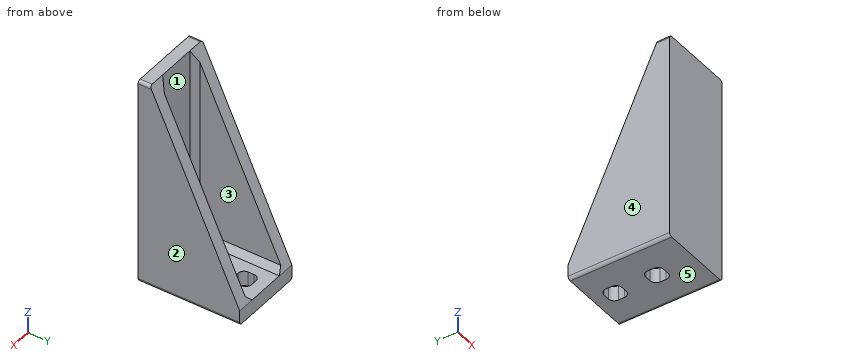
from build123d import *

# Parameters (mm, degrees)
ESBO_O1_W               = 25
ESBO_O1_H               = 70
BASE_DEPTH              = 4
ESBO_O2_W               = 25
ESBO_O2_H               = 5
PAREDE_DO_FUNDO_DEPTH   = 30
PAREDES_START           = -12.5
PAREDES_LATERAIS_DEPTH  = 25
ESBO_O3_W               = 17
ESBO_O3_H               = 30
CORTE_NAS_PAREDES_DEPTH = 65
CHANFRO3_SIZE           = 2
CHANFRO4_SIZE           = 2
CHANFRO5_SIZE           = 2
CHANFRO6_SIZE           = 2
CHANFRO7_SIZE           = 2
PARAFUSO_DEPTH          = 45
FILETE1_R               = 1
FILETE2_R               = 1
FILETE3_R               = 1
FILETE4_R               = 1


with BuildPart() as part:
    # Esboço1 → Base (new body)
    with BuildSketch(Plane(origin=(0, 0, 0), x_dir=(1, 0, 0), z_dir=(0, 1, 0))):
        Rectangle(ESBO_O1_W, ESBO_O1_H)
    extrude(amount=BASE_DEPTH)

    # Esboço2 → Parede do fundo (add)
    with BuildSketch(Plane(origin=(0, 4, 0), x_dir=(1, 0, 0), z_dir=(0, 1, 0))):
        with Locations((0, 32.5)):
            Rectangle(ESBO_O2_W, ESBO_O2_H)
    extrude(amount=PAREDE_DO_FUNDO_DEPTH)

    # Paredes Laterais: read off the stored shape, not the designer's step
    # Paredes Laterais outline → Paredes Laterais (add)
    with BuildSketch(Plane.YZ.offset(PAREDES_START)):
        Polygon((34, -30), (4, 35), (4, -30), align=None)
    extrude(amount=PAREDES_LATERAIS_DEPTH)

    # Esboço3 → Corte nas Paredes (cut)
    with BuildSketch(Plane.XY.offset(35)):
        with Locations((0, 19)):
            Rectangle(ESBO_O3_W, ESBO_O3_H)
    extrude(amount=-CORTE_NAS_PAREDES_DEPTH, mode=Mode.SUBTRACT)

    # Chanfro3
    chanfro3_edges = [part.edges().sort_by_distance(p)[0] for p in [
        (-8.5, 4, 2.5),
    ]]
    chamfer(chanfro3_edges, length=CHANFRO3_SIZE)

    # Chanfro4
    chanfro4_edges = [part.edges().sort_by_distance(p)[0] for p in [
        (8.5, 4, 2.5),
    ]]
    chamfer(chanfro4_edges, length=CHANFRO4_SIZE)

    # Chanfro5
    chanfro5_edges = [part.edges().sort_by_distance(p)[0] for p in [
        (0, 4, -30),
    ]]
    chamfer(chanfro5_edges, length=CHANFRO5_SIZE)

    # Chanfro6
    chanfro6_edges = [part.edges().sort_by_distance(p)[0] for p in [
        (-8.5, 20, -30),
    ]]
    chamfer(chanfro6_edges, length=CHANFRO6_SIZE)

    # Chanfro7
    chanfro7_edges = [part.edges().sort_by_distance(p)[0] for p in [
        (8.5, 20, -30),
    ]]
    chamfer(chanfro7_edges, length=CHANFRO7_SIZE)

    # Esboço4 → Parafuso (cut)
    with BuildSketch(Plane(origin=(0, 0, -35), x_dir=(-1, 0, 0), z_dir=(0, 0, -1))):
        with BuildLine():
            Line((-1, 16), (1, 16))
            ThreePointArc((1, 16), (2.414213562, 15.414213562), (3, 14))
            Line((3, 14), (3, 12))
            ThreePointArc((3, 12), (2.414213562, 10.585786438), (1, 10))
            Line((1, 10), (-1, 10))
            ThreePointArc((-1, 10), (-2.414213562, 10.585786438), (-3, 12))
            Line((-3, 12), (-3, 14))
            ThreePointArc((-3, 14), (-2.414213562, 15.414213562), (-1, 16))
        make_face()
        with BuildLine():
            Line((-3, 26), (-3, 28))
            ThreePointArc((-3, 28), (-2.414213562, 29.414213562), (-1, 30))
            Line((-1, 30), (1, 30))
            ThreePointArc((1, 30), (2.414213562, 29.414213562), (3, 28))
            Line((3, 28), (3, 26))
            ThreePointArc((3, 26), (2.414213562, 24.585786438), (1, 24))
            Line((1, 24), (-1, 24))
            ThreePointArc((-1, 24), (-2.414213562, 24.585786438), (-3, 26))
        make_face()
    extrude(amount=-PARAFUSO_DEPTH, mode=Mode.SUBTRACT)

    # Filete1
    filete1_edges = [part.edges().sort_by_distance(p)[0] for p in [
        (12.5, 17, -35),
    ]]
    fillet(filete1_edges, radius=FILETE1_R)

    # Filete2
    filete2_edges = [part.edges().sort_by_distance(p)[0] for p in [
        (-12.5, 17, -35),
    ]]
    fillet(filete2_edges, radius=FILETE2_R)

    # Filete3
    filete3_edges = [part.edges().sort_by_distance(p)[0] for p in [
        (12.5, 2, 35),
    ]]
    fillet(filete3_edges, radius=FILETE3_R)

    # Filete4
    filete4_edges = [part.edges().sort_by_distance(p)[0] for p in [
        (-12.5, 2, 35),
    ]]
    fillet(filete4_edges, radius=FILETE4_R)


solid = part.part
Geometry: final body of the model. Coordinates: model frame, mm. Face numbers are marked on the shaded views. A direction names the side the tool comes from. Round coordinates to 2 decimals unless told otherwise and drop trailing zeros. Loops run counter-clockwise (first coordinate to the right, second up) from the corner with the lowest first, then second, coordinate; pieces in that order, holes last.
Q1. Section A-A on x = -1.75. Return loops of the section in (y, z), plus the area to 3 significant figures.
Q2. Section D-D on z = -20.5. Return loops of the section in (x, y), plus the area to 3 significant figures.
Q3. Pull-direction query (X, two-part tool) for the marked faces 3, 4 and 5; classes: released by +X, released by -X, zero draft, split by the parting line, or undercut.
Q4. Section C-C on x = 9.75. Return loops of the section in (y, z).
Q5. Section B-B on y = 8.5. Return loops of the section in (x, z).
Q6. Material intervals for L1, parallel to Y at x = 1.25, z = -31; L2, parallel to X at y = 13, z = -1; L3, parallel to Y at x = 5.25, z = -24, sorted ascending.
Q7. Access query for the marked faces 1 and 2. Directions: +Z, -Z, +X, -X, +Y, -Y. A direction counts if a zero-diameter tool reaches every point of the face in a straight line with its end or side. Return the directions, or none.
Q8. Pin query (flat end, axial travel): P1, Ø12, axis at x = 7.5, y = 26, coming from the +Z side; P2, Ø1.6, axis at x = 0.5, z = -31.5, coming from the -Y side; P3, Ø2, axis at x = -7, y = 7, coming from the +Z side; P4, Ø3, axis at x = 3.5, z = -4.5, coming from the +Y side. Return the tip coordinate at first contact, or that it passes through.
Evaluation:
1. outline: (0, -35) - (10.15, -35) - (10.15, -30) - (6, -30) - (4, -28) - (4, 35) - (0, 35) - close; (15.85, -35) - (24.15, -35) - (24.15, -30) - (15.85, -30) - close; (29.85, -35) - (34, -35) - (34, -30) - (29.85, -30) - close
1. area: 375 mm2
2. outline: (-12.5, 0) - (12.5, 0) - (12.5, 29.62) - (8.5, 29.62) - (8.5, 6) - (6.5, 4) - (-6.5, 4) - (-8.5, 6) - (-8.5, 29.62) - (-12.5, 29.62) - close
2. area: 309 mm2
3. face 3: undercut
3. face 4: released by -X
3. face 5: zero draft
4. outline: (0, -35) - (34, -35) - (34, -30) - (4, 35) - (0, 35) - close
5. outline: (-12.5, -34) arc R1 ccw to (-11.5, -35) - (11.5, -35) arc R1 ccw to (12.5, -34) - (12.5, 25.25) - (8.5, 25.25) - (8.5, -28) - (6.5, -30) - (-6.5, -30) - (-8.5, -28) - (-8.5, 25.25) - (-12.5, 25.25) - close
6. L1: y = 0 to 10.02, 15.98 to 24.02, 29.98 to 34
6. L2: x = -12.5 to -8.5, 8.5 to 12.5
6. L3: y = 0 to 4
7. face 1: +Z, +Y
7. face 2: +Z, -Z, +X, +Y, -Y
8. P1: stops at z = 0.15
8. P2: stops at y = 0
8. P3: stops at z = -28.5
8. P4: stops at y = 4
